```python
from build123d import *

# Parameters (mm, degrees)
BOSS_EXTRUDE1_DEPTH      = 2.5
BOSS_EXTRUDE1_DEPTH_BACK = 2.5
CUT_EXTRUDE1_DEPTH       = 1
CUT_EXTRUDE1_DRAFT       = -30
MIRROR1_COPY_1_DEPTH     = 1
MIRROR1_COPY_1_DRAFT     = -30
SKETCH4_R                = 3
CUT_EXTRUDE3_DEPTH       = 26.244307592
SKETCH7_R                = 4
SKETCH7_R_2              = 3
BOSS_EXTRUDE3_DEPTH      = 0.5
SKETCH8_R                = 3
CUT_EXTRUDE4_DEPTH       = 26.348078148
SKETCH9_R                = 4
SKETCH9_R_2              = 3
BOSS_EXTRUDE4_DEPTH      = 0.5
SKETCH10_R               = 0.75
CUT_EXTRUDE5_DEPTH       = 29.56679394
CUT_EXTRUDE5_DEPTH_BACK  = 29.56679394
FILLET1_R                = 0.5
FILLET2_R                = 0.5


with BuildPart() as part:
    # Sketch2 → Boss-Extrude1 (new, two sides)
    with BuildSketch(Plane.XY) as boss_extrude1_sk:
        with BuildLine():
            Line((-15.442222224, -3.67937125), (-6.536442795, -1.557418314))
            ThreePointArc((-6.536442795, -1.557418314), (-5.4304277, -0.851414482), (-5, 0.388118815))
            Line((-5, 0.388118815), (-5, 13.951154424))
            ThreePointArc((-5, 13.951154424), (-4.732050808, 14.951154424), (-4, 15.683205232))
            ThreePointArc((-4, 15.683205232), (0, 16.755002002), (4, 15.683205232))
            ThreePointArc((4, 15.683205232), (4.732050808, 14.951154424), (5, 13.951154424))
            Line((5, 13.951154424), (5, 0.388118815))
            ThreePointArc((5, 0.388118815), (5.4304277, -0.851414482), (6.536442795, -1.557418314))
            Line((6.536442795, -1.557418314), (15.442222224, -3.67937125))
            ThreePointArc((15.442222224, -3.67937125), (16.744432136, -4.68572443), (16.850998146, -6.328021925))
            ThreePointArc((16.850998146, -6.328021925), (0, -18), (-16.850998146, -6.328021925))
            ThreePointArc((-16.850998146, -6.328021925), (-16.744432136, -4.68572443), (-15.442222224, -3.67937125))
        make_face()
    extrude(amount=BOSS_EXTRUDE1_DEPTH)
    extrude(boss_extrude1_sk.sketch, amount=-BOSS_EXTRUDE1_DEPTH_BACK)


with BuildPart() as cut_extrude1_tool:
    # Sketch3 → Cut-Extrude1 (with draft: the straight prism first)
    with BuildSketch(Plane.XY.offset(2.5)):
        with BuildLine():
            ThreePointArc((-13.340399108, -4.720566877), (-14.695107573, -5.833091429), (-14.652958027, -7.585566627))
            ThreePointArc((-14.652958027, -7.585566627), (0, -16.5), (14.652958027, -7.585566627))
            ThreePointArc((14.652958027, -7.585566627), (14.695107573, -5.833091429), (13.340399108, -4.720566877))
            Line((13.340399108, -4.720566877), (4.68940437, -2.659320713))
            ThreePointArc((4.68940437, -2.659320713), (3.722712002, -2.669178372), (2.873576072, -3.131303332))
            ThreePointArc((2.873576072, -3.131303332), (0, -4.25), (-2.873576072, -3.131303332))
            ThreePointArc((-2.873576072, -3.131303332), (-3.722712002, -2.669178372), (-4.68940437, -2.659320713))
            Line((-4.68940437, -2.659320713), (-13.340399108, -4.720566877))
        make_face()
    extrude(amount=-CUT_EXTRUDE1_DEPTH)
    # Cut-Extrude1: the draft: its side faces are tilted about the plane it starts from
    cut_extrude1_sides = [cut_extrude1_tool.faces().sort_by_distance(p)[0] for p in [
        (0, -4.25, 2),
        (-3.722712002, -2.669178372, 2),
        (-9.014901739, -3.689943795, 2),
        (-14.695107573, -5.833091429, 2),
        (0, -16.5, 2),
        (14.695107573, -5.833091429, 2),
        (9.014901739, -3.689943795, 2),
        (3.722712002, -2.669178372, 2),
    ]]
    draft(cut_extrude1_sides, Plane.XY.offset(2.5), CUT_EXTRUDE1_DRAFT)


with BuildPart() as part_1:
    add(part.part)

    # Cut-Extrude1: cut by cut_extrude1_tool
    add(cut_extrude1_tool.part, mode=Mode.SUBTRACT)


with BuildPart() as mirror1_copy_1_tool:
    # Mirror1 copy 1 sketch → Mirror1 copy 1 (with draft: the straight prism first)
    with BuildSketch(Plane(origin=(0, 0, -2.5), x_dir=(1, 0, 0), z_dir=(0, 0, -1))):
        with BuildLine():
            ThreePointArc((-13.340399108, 4.720566877), (-14.695107573, 5.833091429), (-14.652958027, 7.585566627))
            ThreePointArc((-14.652958027, 7.585566627), (0, 16.5), (14.652958027, 7.585566627))
            ThreePointArc((14.652958027, 7.585566627), (14.695107573, 5.833091429), (13.340399108, 4.720566877))
            Line((13.340399108, 4.720566877), (4.68940437, 2.659320713))
            ThreePointArc((4.68940437, 2.659320713), (3.722712002, 2.669178372), (2.873576072, 3.131303332))
            ThreePointArc((2.873576072, 3.131303332), (0, 4.25), (-2.873576072, 3.131303332))
            ThreePointArc((-2.873576072, 3.131303332), (-3.722712002, 2.669178372), (-4.68940437, 2.659320713))
            Line((-4.68940437, 2.659320713), (-13.340399108, 4.720566877))
        make_face()
    extrude(amount=-MIRROR1_COPY_1_DEPTH)
    # Mirror1 copy 1: the draft: its side faces are tilted about the plane it starts from
    mirror1_copy_1_sides = [mirror1_copy_1_tool.faces().sort_by_distance(p)[0] for p in [
        (0, -4.25, -2),
        (-3.722712002, -2.669178372, -2),
        (-9.014901739, -3.689943795, -2),
        (-14.695107573, -5.833091429, -2),
        (0, -16.5, -2),
        (14.695107573, -5.833091429, -2),
        (9.014901739, -3.689943795, -2),
        (3.722712002, -2.669178372, -2),
    ]]
    draft(mirror1_copy_1_sides, Plane(origin=(0, 0, -2.5), x_dir=(1, 0, 0), z_dir=(0, 0, -1)), MIRROR1_COPY_1_DRAFT)


with BuildPart() as part_2:
    add(part_1.part)

    # Mirror1 copy 1: cut by mirror1_copy_1_tool
    add(mirror1_copy_1_tool.part, mode=Mode.SUBTRACT)

    # Sketch4 → Cut-Extrude3 (cut, through all)
    with BuildSketch(Plane.XY.offset(2.5)):
        Circle(SKETCH4_R)
    extrude(amount=-CUT_EXTRUDE3_DEPTH, mode=Mode.SUBTRACT)

    # Sketch7 → Boss-Extrude3 (add)
    with BuildSketch(Plane(origin=(0, 0, -2.5), x_dir=(-1, 0, 0), z_dir=(0, 0, -1))):
        Circle(SKETCH7_R)
        with Locations(Location((0, 0, 0), (0, 0, 180))):
            Circle(SKETCH7_R_2, mode=Mode.SUBTRACT)
    extrude(amount=BOSS_EXTRUDE3_DEPTH)

    # Sketch8 → Cut-Extrude4 (cut, through all)
    with BuildSketch(Plane.XY.offset(2.5)):
        with Locations((0, 9)):
            Circle(SKETCH8_R)
    extrude(amount=-CUT_EXTRUDE4_DEPTH, mode=Mode.SUBTRACT)

    # Sketch9 → Boss-Extrude4 (add)
    with BuildSketch(Plane.XY.offset(2.5)):
        with Locations(Location((0, 9, 0), (0, 0, 180))):
            Circle(SKETCH9_R)
        with Locations((0, 9)):
            Circle(SKETCH9_R_2, mode=Mode.SUBTRACT)
    extrude(amount=BOSS_EXTRUDE4_DEPTH)

    # Sketch10 → Cut-Extrude5 (cut, two sides)
    with BuildSketch(Plane.ZY.offset(5)) as cut_extrude5_sk:
        with Locations((0, 9)):
            Circle(SKETCH10_R)
        Circle(SKETCH10_R)
    extrude(amount=CUT_EXTRUDE5_DEPTH, mode=Mode.SUBTRACT)
    extrude(cut_extrude5_sk.sketch, amount=-CUT_EXTRUDE5_DEPTH_BACK, mode=Mode.SUBTRACT)

    # Fillet1
    fillet1_edges = [part_2.edges().sort_by_distance(p)[0] for p in [
        (-3.867954613, -3.227960903, 1.5),
        (8.8810843, -4.251571987, 1.5),
        (14.170219486, -6.073561446, 1.5),
        (0, -15.922649731, 1.5),
        (-14.170219486, -6.073561446, 1.5),
        (-8.8810843, -4.251571987, 1.5),
        (0, -4.827350269, 1.5),
        (3.867954613, -3.227960903, 1.5),
    ]]
    fillet(fillet1_edges, radius=FILLET1_R)

    # Fillet2
    fillet2_edges = [part_2.edges().sort_by_distance(p)[0] for p in [
        (-14.170219486, -6.073561446, -1.5),
        (3.867954613, -3.227960903, -1.5),
        (0, -4.827350269, -1.5),
        (-8.8810843, -4.251571987, -1.5),
        (0, -15.922649731, -1.5),
        (14.170219486, -6.073561446, -1.5),
        (8.8810843, -4.251571987, -1.5),
        (-3.867954613, -3.227960903, -1.5),
    ]]
    fillet(fillet2_edges, radius=FILLET2_R)


solid = part_2.part
```
The model under review builds one solid part; all positions refer to its coordinate system, in mm. A direction names the side the tool comes from. Coordinates: 2 decimals unless noted, no trailing zeros. Order: outer loops, then holes, each group sorted by start corner. A loop starts at its lowest first (then second) coordinate and runs counter-clockwise, first axis right, second up. Notation, with made-up numbers: (88, 47) -> (98, 47) arc R18 ccw to (98, 71) -> close; hole circle Ø11 at (55, -20). An arc over 180 degrees is marked (long way). Answer in a Markdown table with one row per item. Add a question column.
Item 1: Machinability: for faces 1 (the flat face through (9.026, -3.912, 2.13)), 2 (the flat face through (-5, 7, 0)), 3 (the flat face through (-1, 6, 3)), which of the approach directions +Z, -Z, +X, -X, +Y, -Y give a long, thin tool a straight path to every point of the face, cutting with its end or side? Answer none if there is none.
Item 2: Mouldability with a two-part tool opening along Y and no side actions: class faces 4 (the flat face through (-8.9, -3.9, -2.1)), 5 (the flat face through (3, 3, -2.5)), 6 (the cylindrical face through (2.86, -0.9, -0.21)), 7 (the cylindrical face through (4.725, 14.964, 0.035)) as +Y half, -Y half, draft (parallel to the pull), parting line (faces both ways), or undercut.
Item 3: Clearance check with flat-ended pins moving along their axes: pin 1 (1.4 mm diameter, centred on y = 9, z = 0, fed in from -X); pin 2 (2 mm diameter, centred on y = 0, z = 0, fed in from +X); pin 3 (8 mm diameter, centred on x = 0, y = 9, fed in from -Z); pin 4 (2 mm diameter, centred on x = 13, z = -1, fed in from -Y). State where each tip first meets the part, or that it passes through.
Item 4: To check wall thickness, follow probe 1 along Y at (x, z) = (0, -0.7) (3 decimals); probe 2 along Y at (x, z) = (-2, 2); probe 3 along Z at (x, y) = (5.5, -4). State the ranges of each line that lie inside material, in increasing order.
Item 5: We need section B-B on z = 0. Write out the cut boundary in (x, y) (3 decimals).
Item 6: We need section D-D on y = -2. Write out the cut boundary in (x, z), plus the area to 3 significant figures.
Item 7: We need section A-A on y = 9. Write out the cut boundary in (x, z).
Item 8: We need section C-C on x = 0. Give the number of separate pieces and of enclosed holes in the cut face, plus the area to 3 significant figures.
Final values:
| question | item | result |
|---|---|---|
| 1 | face 1 | +Z |
| 1 | face 2 | +Z, -Z, -X, +Y |
| 1 | face 3 | +Z, +X, -X, +Y, -Y |
| 2 | face 4 | undercut |
| 2 | face 5 | draft |
| 2 | face 6 | undercut |
| 2 | face 7 | +Y half |
| 3 | pin 1 | passes through |
| 3 | pin 2 | stops at x = 5.56 |
| 3 | pin 3 | stops at z = -2.5 |
| 3 | pin 4 | stops at y = -13.42 |
| 4 | probe 1 | y = -18 to -3, 3 to 6, 12 to 16.755 |
| 4 | probe 2 | y = -17.89 to -16.09, -4.07 to -2.24, 2.24 to 6.76, 11.24 to 16.5 |
| 4 | probe 3 | z = -1.5 to 1.5 |
| 5 | outline | (-16.851, -6.328) arc R18 ccw to (16.851, -6.328) arc R2 ccw to (15.442, -3.679) -> (6.536, -1.557) arc R2 cw to (5.355, -0.75) -> (2.905, -0.75) arc R3 cw to (-2.905, -0.75) -> (-5.355, -0.75) arc R2 cw to (-6.536, -1.557) -> (-15.442, -3.679) arc R2 ccw to start; (-5, 0.75) -> (-2.905, 0.75) arc R3 cw to (2.905, 0.75) -> (5, 0.75) -> (5, 8.25) -> (2.905, 8.25) arc R3 cw to (-2.905, 8.25) -> (-5, 8.25) -> close; (-5, 9.75) -> (-2.905, 9.75) arc R3 cw to (2.905, 9.75) -> (5, 9.75) -> (5, 13.951) arc R2 ccw to (4, 15.683) arc R8 ccw to (-4, 15.683) arc R2 ccw to (-5, 13.951) -> close |
| 6 | outline | (-8.39, -2.5) -> (-3.46, -2.5) -> (-3.46, -3) -> (-2.24, -3) -> (-2.24, 2.5) -> (-8.39, 2.5) -> close; (2.24, -3) -> (3.46, -3) -> (3.46, -2.5) -> (8.39, -2.5) -> (8.39, 2.5) -> (2.24, 2.5) -> close |
| 6 | area | 62.8 mm2 |
| 7 | outline | (-5, -2.5) -> (-3, -2.5) -> (-3, -0.75) -> (-5, -0.75) -> close; (-5, 0.75) -> (-3, 0.75) -> (-3, 3) -> (-4, 3) -> (-4, 2.5) -> (-5, 2.5) -> close; (3, -2.5) -> (5, -2.5) -> (5, -0.75) -> (3, -0.75) -> close; (3, 0.75) -> (5, 0.75) -> (5, 2.5) -> (4, 2.5) -> (4, 3) -> (3, 3) -> close |
| 8 | separate pieces | 3 |
| 8 | enclosed holes | 0 |
| 8 | area | 92.5 mm2 |
